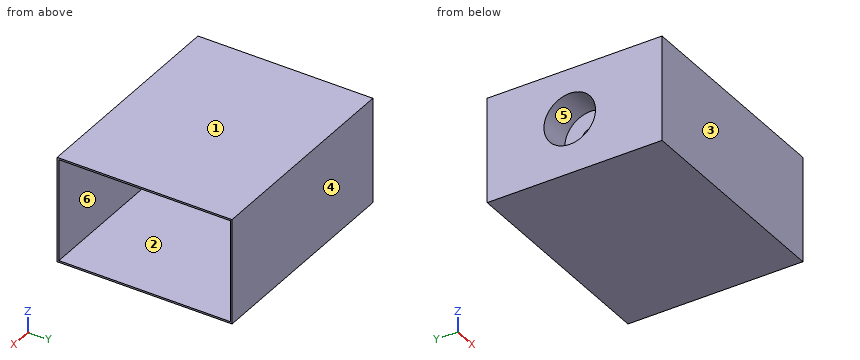
from build123d import *

# Parameters (mm, degrees)
F0_W     = 118.9471073449
F0_H     = 24.972319603
F2_W     = 255.0741881132
F2_H     = 153.8173779845
F3_DEPTH = 213.868
F4_DEPTH = 105.664
F5_T     = -2.54


with BuildPart() as f1:
    # F0 (on Top) → F1 (revolve)
    with BuildSketch(Plane.XY):
        with Locations((1.3143327087, 25.1366123557)):
            Rectangle(F0_W, F0_H)
    revolve(axis=Axis((7.0028230548, 0, 0), (-1, 0, 0)))

    # F2 (on Right) → F3 (join)
    with BuildSketch(Plane.YZ):
        with Locations((-7.0527419448, -3.2536052167)):
            Rectangle(F2_W, F2_H)
    extrude(amount=F3_DEPTH)

    # F4 (add): a face of the model
    f4_faces = [f1.faces().sort_by_distance(p)[0] for p in [
        (0, 117.50571774, -3.2536052167),
    ]]
    extrude(f4_faces, amount=F4_DEPTH)

    # F5
    f5_openings = [f1.faces().sort_by_distance(p)[0] for p in [
        (213.868, -7.052742, -3.253605),
    ]]
    offset(amount=F5_T, openings=f5_openings, kind=Kind.INTERSECTION)


solid = f1.part
CAD build for the part. Positions are in the model's coordinates, mm. Face numbers are marked on the shaded views. A direction names the side the tool comes from. Round coordinates to 2 decimals unless told otherwise and drop trailing zeros. Loops run counter-clockwise (first coordinate to the right, second up) from the corner with the lowest first, then second, coordinate; pieces in that order, holes last.
(1) Wall check: line 1 along Z through (x, y) = (-73.5, 0); line 2 along Z through (x, y) = (-64, -1); line 3 along Y through (x, z) = (150, 42). Give the ranges that are in metal, low to high.
(2) Which spindle directions (+Z, -Z, +X, -X, +Y, -Y) get a long thin tool onto all of the face, cutting with end or side? Do the marked faces 4, 5 and 6. Say none if no direction does.
(3) Cut at D-D (z = 0). Give the cut face in (x, y), plus the area to 3 significant figures.
(4) Cut at C-C (x = 69). Give the cut face in (y, z).
(5) Cut at B-B (y = -81.5). Give the cut face in (x, z), plus the area to 3 significant figures.
(6) Cut at A-A (z = -49). Give the cut face in (x, y), plus the area to 3 significant figures.
(7) Two-plate mould, pull along Z, no slides. Class the marked faces 1, 2 and 3: +Z half, -Z half, draft (parallel to the pull), parting line (faces both ways), or undercut.
(8) Drop flat-ended pins along their axis: pin 1 (12 mm diameter, centred on y = 40.5, z = 17, fed in from +X); pin 2 (24 mm diameter, centred on y = -14.5, z = -16, fed in from +X); pin 3 (20 mm diameter, centred on y = 0, z = 0, fed in from -X). Give the stop position or say it passes through.
Findings below:
1. line 1: z = -80.16 to -77.62, -40.16 to -37.62, 37.62 to 40.16, 71.12 to 73.66
1. line 2: z = -80.16 to -77.62, -40.15 to -37.61, 37.61 to 40.15, 71.12 to 73.66
1. line 3: y = -134.59 to -132.05, 117.94 to 120.48
2. face 4: +Z, -Z, +X, -X, +Y
2. face 5: -X
2. face 6: +X
3. outline: (-105.66, -134.59) - (213.87, -134.59) - (213.87, -132.05) - (-103.12, -132.05) - (-103.12, -40.16) - (-55.62, -40.16) - (-55.62, -15.19) - (2.54, -15.19) - (2.54, 15.19) - (-55.62, 15.19) - (-55.62, 40.16) - (-103.12, 40.16) - (-103.12, 117.94) - (213.87, 117.94) - (213.87, 120.48) - (-105.66, 120.48) - (-105.66, 37.62) - (-58.16, 37.62) - (-58.16, 12.65) - (0, 12.65) - (0, -12.65) - (-58.16, -12.65) - (-58.16, -37.62) - (-105.66, -37.62) - close
3. area: 2,790 mm2
4. outline: (-134.59, -80.16) - (120.48, -80.16) - (120.48, 73.66) - (-134.59, 73.66) - close; hole (-132.05, -77.62) - (117.94, -77.62) - (117.94, 71.12) - (-132.05, 71.12) - close
5. outline: (-105.66, -80.16) - (213.87, -80.16) - (213.87, -77.62) - (-103.12, -77.62) - (-103.12, 71.12) - (213.87, 71.12) - (213.87, 73.66) - (-105.66, 73.66) - close
5. area: 2,000 mm2
6. outline: (-105.66, -134.59) - (213.87, -134.59) - (213.87, -132.05) - (-103.12, -132.05) - (-103.12, 117.94) - (213.87, 117.94) - (213.87, 120.48) - (-105.66, 120.48) - close
6. area: 2,260 mm2
7. face 1: +Z half
7. face 2: undercut
7. face 3: draft
8. pin 1: stops at x = -55.62
8. pin 2: stops at x = 2.54
8. pin 3: stops at x = 0
